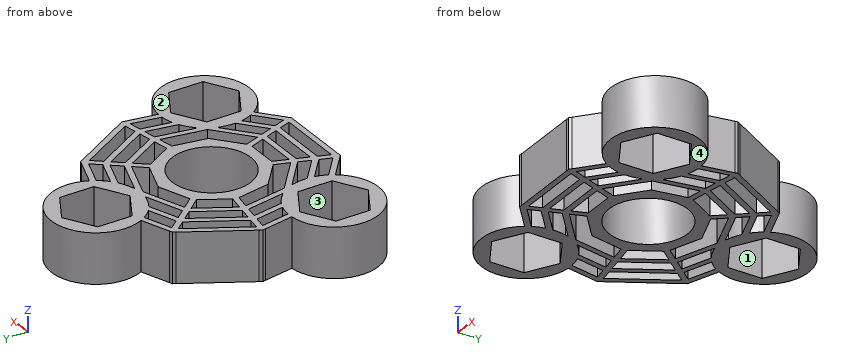
from build123d import *

# Parameters (mm, degrees)
F0_R     = 12.5
F1_DEPTH = 14
F0_R_2   = 11.025
F2_COUNT = 3
F4_DEPTH = 14
F5_COUNT = 3


# Not quite as in the source:
# - a feature names something its author has since deleted; it is built from what else it names


with BuildPart() as f1:
    # F0 (on Top) → F1 (new body)
    with BuildSketch(Plane.XY):
        with Locations((0, 32.5)):
            Circle(F0_R)
        Polygon((8.3354945114, 37.3125), (8.3354945114, 27.6875), (0, 22.875), (-8.3354945114, 27.6875), (-8.3354945114, 37.3125), (0, 42.125), align=None, mode=Mode.SUBTRACT)
    extrude(amount=F1_DEPTH)


with BuildPart() as f1b:
    # F0 (on Top) → F1, piece 2 (new body)
    with BuildSketch(Plane.XY):
        Polygon((9.6418141453, 11.4906666468), (0, 15), (-9.6418141453, 11.4906666468), (-14.7721162952, 2.604722665), (-12.9903810568, -7.5), (-5.1303021499, -14.0953893118), (5.1303021499, -14.0953893118), (12.9903810568, -7.5), (14.7721162952, 2.604722665), align=None)
        Circle(F0_R_2, mode=Mode.SUBTRACT)
    extrude(amount=F1_DEPTH)


with BuildPart() as f2_1:
    # F2: instance of F1
    add(f1.part.rotate(Axis((0, 0, 0), (0, 0, -1)), 1 * 360 / F2_COUNT))


with BuildPart() as f2_2:
    # F2: instance of F1
    add(f1.part.rotate(Axis((0, 0, 0), (0, 0, -1)), 2 * 360 / F2_COUNT))


with BuildPart() as f1_1:
    add(f1.part)

    add(f1b.part)  # F4 merges F1b

    add(f2_2.part)  # F4 merges F2_2
    # F3 (on Top) → F4 (join, through all)
    with BuildSketch(Plane.XY):
        Polygon((-14.3464451862, 3.3420066531), (-18.5384872699, 4.0811767767), (-18.9641583789, 3.3438927886), (-18.8163243541, 2.5054843719), (-14.6242822705, 1.7663142483), (-14.7721162952, 2.604722665), align=None)
        Polygon((-8.8418141453, 11.7818428342), (-11.5779752919, 15.0426727106), (-12.3779752919, 14.7514965232), (-12.8036464009, 14.0142125351), (-10.0674852543, 10.7533826587), (-9.6418141453, 11.4906666468), align=None)
        Polygon((-18.9641583789, 3.3438927886), (-18.5384872699, 4.0811767767), (-20.2153041033, 4.3768448262), (-20.6409752123, 3.6395608381), (-20.4931411876, 2.8011524213), (-18.8163243541, 2.5054843719), align=None)
        Polygon((-12.3779752919, 14.7514965232), (-11.5779752919, 15.0426727106), (-12.6724397505, 16.3470046611), (-13.4724397505, 16.0558284737), (-13.8981108595, 15.3185444856), (-12.8036464009, 14.0142125351), align=None)
        Polygon((-13.4724397505, 16.0558284737), (-12.6724397505, 16.3470046611), (-14.8613686678, 18.9556685622), (-15.6613686678, 18.6644923748), (-16.0870397768, 17.9272083867), (-13.8981108595, 15.3185444856), align=None)
        Polygon((-20.6409752123, 3.6395608381), (-20.2153041033, 4.3768448262), (-23.5689377703, 4.968180925), (-23.9946088793, 4.230896937), (-23.8467748545, 3.3924885202), (-20.4931411876, 2.8011524213), align=None)
        Polygon((-23.5689377703, 4.968180925), (-25.2457546037, 5.2638489745), (-25.6714257127, 4.5265649864), (-25.523591688, 3.6881565697), (-23.8467748545, 3.3924885202), (-23.9946088793, 4.230896937), align=None)
        Polygon((-14.8613686678, 18.9556685622), (-15.9558331265, 20.2600005128), (-16.7558331265, 19.9688243254), (-17.1815042355, 19.2315403373), (-16.0870397768, 17.9272083867), (-15.6613686678, 18.6644923748), align=None)
        Polygon((-15.9558331265, 20.2600005128), (-18.1447620438, 22.8686644139), (-18.9447620438, 22.5774882265), (-19.3704331527, 21.8402042384), (-17.1815042355, 19.2315403373), (-16.7558331265, 19.9688243254), align=None)
        Polygon((-25.2457546037, 5.2638489745), (-28.5993882707, 5.8551850734), (-29.0250593797, 5.1179010853), (-28.8772253549, 4.2794926686), (-25.523591688, 3.6881565697), (-25.6714257127, 4.5265649864), align=None)
        Polygon((-28.5993882707, 5.8551850734), (-30.2762051041, 6.1508531228), (-30.7018762131, 5.4135691347), (-30.5540421884, 4.575160718), (-28.8772253549, 4.2794926686), (-29.0250593797, 5.1179010853), align=None)
        Polygon((-18.1447620438, 22.8686644139), (-19.2392265024, 24.1729963645), (-20.0392265024, 23.881820177), (-20.4648976114, 23.144536189), (-19.3704331527, 21.8402042384), (-18.9447620438, 22.5774882265), align=None)
        with BuildLine():
            ThreePointArc((-10.4650421032, 25.6638538798), (-10.8865068143, 26.3572018279), (-11.262100915, 27.0764326333))
            Line((-11.262100915, 27.0764326333), (-19.2392265024, 24.1729963645))
            Line((-19.2392265024, 24.1729963645), (-18.1447620438, 22.8686644139))
            Line((-18.1447620438, 22.8686644139), (-10.4650421032, 25.6638538798))
        make_face()
        Polygon((-19.3704331527, 21.8402042384), (-20.4648976114, 23.144536189), (-30.2762051041, 6.1508531228), (-28.5993882707, 5.8551850734), align=None)
        Polygon((-16.0870397768, 17.9272083867), (-17.1815042355, 19.2315403373), (-25.2457546037, 5.2638489745), (-23.5689377703, 4.968180925), align=None)
        with BuildLine():
            ThreePointArc((-6.6788350915, 21.9338672249), (-7.4683996582, 22.4763775737), (-8.2140988038, 23.0777613678))
            Line((-8.2140988038, 23.0777613678), (-15.9558331265, 20.2600005128))
            Line((-15.9558331265, 20.2600005128), (-14.8613686678, 18.9556685622))
            Line((-14.8613686678, 18.9556685622), (-6.6788350915, 21.9338672249))
        make_face()
        with BuildLine():
            Line((-11.5779752919, 15.0426727106), (3.1518577067, 20.4038934778))
            ThreePointArc((3.1518577067, 20.4038934778), (0.5214979159, 20.0108831408), (-2.1324694589, 20.1832401173))
            Line((-2.1324694589, 20.1832401173), (-12.6724397505, 16.3470046611))
            Line((-12.6724397505, 16.3470046611), (-11.5779752919, 15.0426727106))
        make_face()
        Polygon((-18.5384872699, 4.0811767767), (-12.8036464009, 14.0142125351), (-13.8981108595, 15.3185444856), (-20.2153041033, 4.3768448262), align=None)
        with BuildLine():
            Line((-28.8772253549, 4.2794926686), (-30.5540421884, 4.575160718))
            Line((-30.5540421884, 4.575160718), (-29.0799289618, -3.7849508243))
            ThreePointArc((-29.0799289618, -3.7849508243), (-28.2692597628, -3.7506094543), (-27.4580704705, -3.7689346268))
            Line((-27.4580704705, -3.7689346268), (-28.8772253549, 4.2794926686))
        make_face()
        with BuildLine():
            Line((-23.8467748545, 3.3924885202), (-25.523591688, 3.6881565697))
            Line((-25.523591688, 3.6881565697), (-24.0929770089, -4.4252624506))
            ThreePointArc((-24.0929770089, -4.4252624506), (-23.199313793, -4.7703649572), (-22.3347037658, -5.1828927555))
            Line((-22.3347037658, -5.1828927555), (-23.8467748545, 3.3924885202))
        make_face()
        with BuildLine():
            Line((-16.0943612345, -12.931535582), (-18.8163243541, 2.5054843719))
            Line((-18.8163243541, 2.5054843719), (-20.4931411876, 2.8011524213))
            Line((-20.4931411876, 2.8011524213), (-18.5454334017, -8.2448473345))
            ThreePointArc((-18.5454334017, -8.2448473345), (-17.0691841941, -10.4570720136), (-16.0943612345, -12.931535582))
        make_face()
    extrude(amount=F4_DEPTH)



with BuildPart() as f1_2:
    add(f1_1.part)

    add(f2_1.part)  # F5 merges F2_1
    # F5: F1 ×3 about axis
    f5_axis = Axis((0, 0, 0), (0, 0, -1))
    for i in range(1, F5_COUNT):
        add(f1_1.part.rotate(f5_axis, i * 360 / F5_COUNT))


solid = f1_2.part
Source: CAD feature listing. Evaluate the final solid. Frame: model axes, mm. Face numbers are marked on the shaded views. A direction names the side the tool comes from. Round coordinates to 2 decimals unless told otherwise and drop trailing zeros. Loops run counter-clockwise (first coordinate to the right, second up) from the corner with the lowest first, then second, coordinate; pieces in that order, holes last. Notation, with made-up numbers: (5, 37.5) - (21, 37.5) arc R19 ccw to (21, 43.5) - close; hole circle Ø4 at (13, 42.25). An arc over 180 degrees is marked (long way). Write item = value, one per line. Start each with the question number.
Item 1: Material intervals for line 1 (Y direction, x = -36, z = 4.5); line 2 (X direction, y = 38.5, z = 3.75); line 3 (Y direction, x = 34, z = 8.5), sorted ascending.
Item 2: Section query A-A on y = 33. Output: boundary loops of the cut face in (x, z), plus the area to 3 significant figures.
Item 3: Section query B-B on y = -2. Count the separate pieces of the cut face and the enclosed holes in it, plus the area to 3 significant figures.
Item 4: Mould query, pull axis Y, two halves, no side actions, for the marked faces 1 and 2. Classes: released by +Y, released by -Y, zero draft, split by the parting line, or undercut.
Item 5: Reachability of the marked faces 3 and 4 from +Z, -Z, +X, -X, +Y, -Y: full face, straight path, thin tool, end or side. Return the list, or none.
Item 6: First-contact query: pin 1 Ø5 at (y, z) = (15.5, 7) entering from +X; pin 2 Ø8 at (x, z) = (23, 2) entering from -Y; pin 3 Ø3 at (y, z) = (31, 9.5) entering from -X; pin 4 Ø17.5 at (x, y) = (0, 0) entering from -Z. Flat tips, straight axial feed; report the tip coordinate or a pass-through.
Results list:
q1.line_1 = -25.97 to -21.34, -11.16 to -6.53
q1.line_2 = -10.97 to -6.28, 6.28 to 10.97
q1.line_3 = -27.29 to -22.5, -10 to -5.21
q2.outline = (-12.49, 0) - (-8.34, 0) - (-8.34, 14) - (-12.49, 14) - close; (8.34, 0) - (12.49, 0) - (12.49, 14) - (8.34, 14) - close
q2.area = 116 mm²
q3.separate_pieces = 8
q3.enclosed_holes = 0
q3.area = 224 mm²
q4.face_1 = undercut
q4.face_2 = zero draft
q5.face_3 = +Z, -Z
q5.face_4 = -Z, +X, -X, +Y, -Y
q6.pin_1 = 26.32
q6.pin_2 = -28.7
q6.pin_3 = -12.5
q6.pin_4 = through
